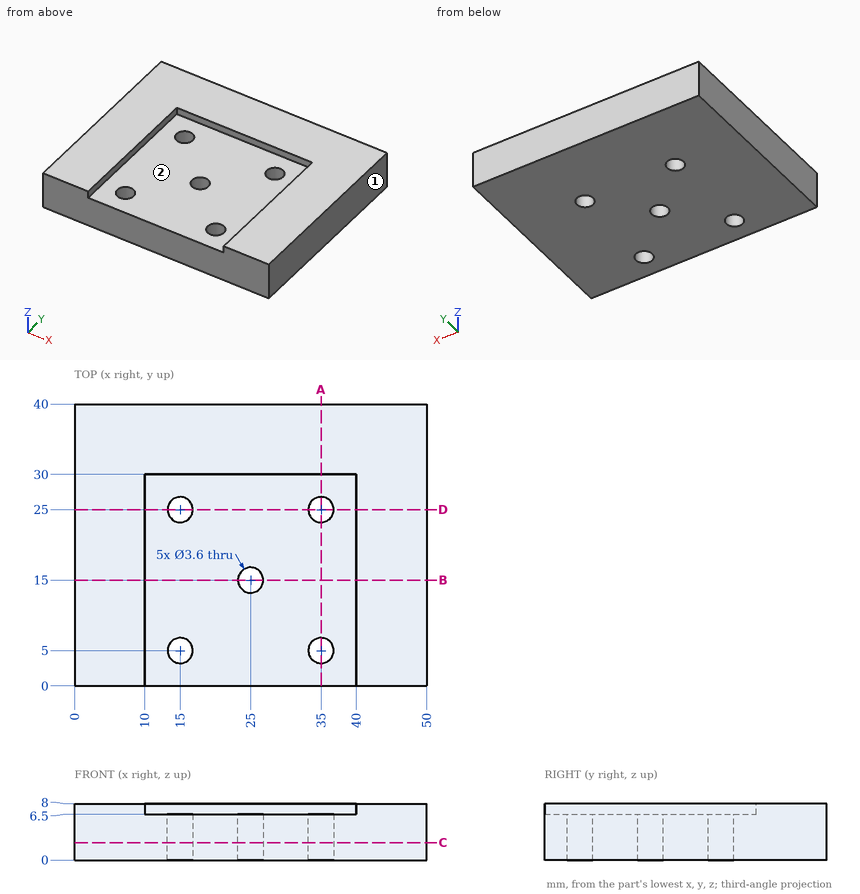
Here's the drawing with two shaded views (mm, measured from the low corner). I have some questions. A direction names the side the tool comes from. Coordinates: 2 decimals unless noted, no trailing zeros. Loops run counter-clockwise (first coordinate to the right, second up) from the corner with the lowest first, then second, coordinate; pieces in that order, holes last. Notation, with made-up numbers: (-10, 34.5) -> (45, 34.5) arc R24 cw to (45, 50.5) -> close; hole circle Ø11 at (-2, 86.5). An arc over 180 degrees is marked (long way). Use one line per item in the form item = value. Start each with the question number.
(1) Please list where these lines run through material, in increasing order: line 1 along Y through (x, z) = (15, 4.5); line 2 along X through (y, z) = (4.5, 0.5); line 3 along X through (y, z) = (8, 7).
(2) On a 3-axis mill with a long thin cutter (end or side, diameter ignored), from which of +Z, -Z, +X, -X, +Y, -Y can I reach the whole of each face in a straight line? I mean the marked faces 1 and 2. Say none if no direction works.
(3) If we section it at C-C (z = 2.5): Please give me the cut outline in (x, y), then the cut area to 3 significant figures.
(4) If we section it at A-A (x = 35): Please give me the cut outline in (y, z).
(5) If we section it at B-B (y = 15): Please give me the cut outline in (x, z).
(6) Will these pins go through, and if not, where does the flat tip stop? pin 1 (1 mm diameter, centred on x = 40.5, y = 34.5, fed in from -Z); pin 2 (9 mm diameter, centred on x = 20, y = 17.5, fed in from +Z); pin 3 (2 mm diameter, centred on x = 15, y = 25, fed in from -Z).
(7) If we section it at D-D (y = 25): Please give me the cut outline in (x, z), then the cut area to 3 significant figures.
Verdict:
q1.line_1 = 0 to 3.2, 6.8 to 23.2, 26.8 to 40
q1.line_2 = 0 to 13.27, 16.73 to 33.27, 36.73 to 50
q1.line_3 = 0 to 10, 40 to 50
q2.face_1 = +Z, -Z, +X, +Y, -Y
q2.face_2 = +Z, -Y
q3.outline = (0, 0) -> (50, 0) -> (50, 40) -> (0, 40) -> close; hole circle Ø3.6 at (15, 5); hole circle Ø3.6 at (15, 25); hole circle Ø3.6 at (25, 15); hole circle Ø3.6 at (35, 5); hole circle Ø3.6 at (35, 25)
q3.area = 1,950 mm²
q4.outline = (0, 0) -> (3.2, 0) -> (3.2, 6.5) -> (0, 6.5) -> close; (6.8, 0) -> (23.2, 0) -> (23.2, 6.5) -> (6.8, 6.5) -> close; (26.8, 0) -> (40, 0) -> (40, 8) -> (30, 8) -> (30, 6.5) -> (26.8, 6.5) -> close
q5.outline = (0, 0) -> (23.2, 0) -> (23.2, 6.5) -> (10, 6.5) -> (10, 8) -> (0, 8) -> close; (26.8, 0) -> (50, 0) -> (50, 8) -> (40, 8) -> (40, 6.5) -> (26.8, 6.5) -> close
q6.pin_1 = 0
q6.pin_2 = 6.5
q6.pin_3 = through
q7.outline = (0, 0) -> (13.2, 0) -> (13.2, 6.5) -> (10, 6.5) -> (10, 8) -> (0, 8) -> close; (16.8, 0) -> (33.2, 0) -> (33.2, 6.5) -> (16.8, 6.5) -> close; (36.8, 0) -> (50, 0) -> (50, 8) -> (40, 8) -> (40, 6.5) -> (36.8, 6.5) -> close
q7.area = 308 mm²
